Model file for the job. Use its own axes, mm. Face numbers are marked on the shaded views. A direction names the side the tool comes from. Give positions to 0.01 mm unless a question says otherwise; leave off trailing zeros. Order: outer loops, then holes, each group sorted by start corner. A loop starts at its lowest first (then second) coordinate and runs counter-clockwise, first axis right, second up. Notation, with made-up numbers: (25, 69.25) -> (68, 69.25) arc R20 ccw to (68, 92.25) -> close; hole circle Ø11 at (39.25, 86). An arc over 180 degrees is marked (long way). Answer in a Markdown table with one row per item. Add a question column.
from build123d import *

# Parameters (mm, degrees)
EXTRUDE_THIN1_DEPTH        = 12.7
FILLET1_R                  = 12.7
SKETCH2_R                  = 3.9624
CUT_EXTRUDE1_DEPTH         = 71.952548404
F_31_0_12_DIAMETER_HOLE1_D = 3.048


with BuildPart() as part:
    # Sketch1 → Extrude-Thin1 (new, symmetric)
    with BuildSketch(Plane.XY):
        with BuildLine():
            Line((-26.035, -64.77), (-26.035, -3.9624))
            ThreePointArc((-26.035, -3.9624), (-24.87443991, -1.16056009), (-22.0726, 0))
            Line((-22.0726, 0), (22.0726, 0))
            ThreePointArc((22.0726, 0), (24.87443991, -1.16056009), (26.035, -3.9624))
            Line((26.035, -3.9624), (26.035, -64.77))
            Line((26.035, -64.77), (23.876, -64.77))
            Line((23.876, -64.77), (23.876, -3.9624))
            ThreePointArc((23.876, -3.9624), (23.347796369, -2.687203631), (22.0726, -2.159))
            Line((22.0726, -2.159), (-22.0726, -2.159))
            ThreePointArc((-22.0726, -2.159), (-23.347796369, -2.687203631), (-23.876, -3.9624))
            Line((-23.876, -3.9624), (-23.876, -64.77))
            Line((-23.876, -64.77), (-26.035, -64.77))
        make_face()
    extrude(amount=EXTRUDE_THIN1_DEPTH, both=True)

    # Fillet1
    fillet1_edges = [part.edges().sort_by_distance(p)[0] for p in [
        (24.9555, -64.77, -12.7),
        (24.9555, -64.77, 12.7),
        (-24.9555, -64.77, -12.7),
        (-24.9555, -64.77, 12.7),
    ]]
    fillet(fillet1_edges, radius=FILLET1_R - 0.0001)  # a hair under: the kernel refuses the full size

    # Sketch2 → Cut-Extrude1 (cut, through all)
    with BuildSketch(Plane(origin=(0, 0, 0), x_dir=(1, 0, 0), z_dir=(0, 1, 0))):
        with Locations(Location((0, 0, 0), (0, 0, 270))):
            Circle(SKETCH2_R)
    extrude(amount=-CUT_EXTRUDE1_DEPTH, mode=Mode.SUBTRACT)

    # #31 (0.12) Diameter Hole1 (through all)
    with Locations(Plane(origin=(0, 0, 0), x_dir=(1, 0, 0), z_dir=(0, 1, 0))):
        with Locations((0, -7.112), (0, 7.112), (-7.112, 0), (7.112, 0), (18.6309, 0), (-18.6309, 0)):
            Hole(F_31_0_12_DIAMETER_HOLE1_D / 2)


solid = part.part
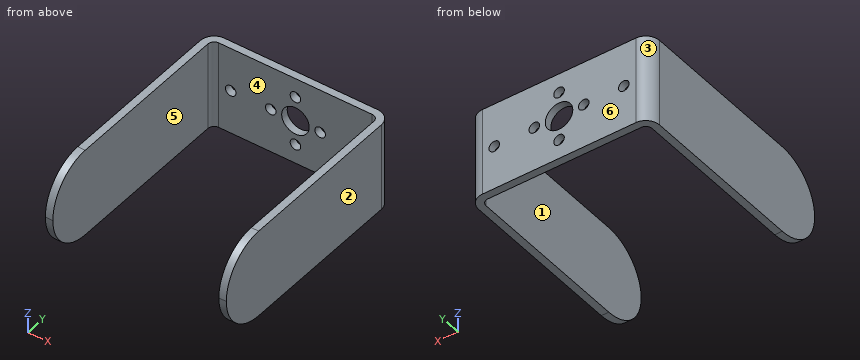
Item 1: Saw through at B-B on y = -21. List the corners of the cut face in (x, z) (3 decimals), plus the area to 3 significant figures.
Item 2: Two-plate mould, pull along X, no slides. Class the marked faces 1, 2, 3 and 4: pulls with the +X half, pulls with the -X half, needs draft (parallel to the pull), parting line crosses it, or undercut.
Item 3: Saw through at C-C on z = 10. List the corners of the cut face in (x, y) (3 decimals).
Item 4: Saw through at A-A on x = 0. List the corners of the cut face in (y, z), plus the area to 3 significant figures.
Item 5: Pin check, flat tips, straight feed: pin 1 Ø4 at (x, z) = (7.112, 0) entering from -Y; pin 2 Ø2.5 at (x, z) = (0, 7.112) entering from +Y. Stop position of each tip, or through.
Item 6: Wall check: line 1 (X direction, y = -26, z = 10.75) (3 decimals); line 2 (Y direction, x = 8.5, z = 5.5); line 3 (X direction, y = -3.5, z = 10.5). Give the ranges that are in metal, low to high.
Item 7: Which spindle directions (+Z, -Z, +X, -X, +Y, -Y) get a long thin tool onto all of the face, cutting with end or side? Do the marked faces 5 and 6. Say none if no direction does.
Evaluation:
| question | item | result |
|---|---|---|
| 1 | outline | (-26.035, -12.7) -> (-23.876, -12.7) -> (-23.876, 12.7) -> (-26.035, 12.7) -> close; (23.876, -12.7) -> (26.035, -12.7) -> (26.035, 12.7) -> (23.876, 12.7) -> close |
| 1 | area | 110 mm2 |
| 2 | face 1 | undercut |
| 2 | face 2 | pulls with the +X half |
| 2 | face 3 | pulls with the -X half |
| 2 | face 4 | undercut |
| 3 | outline | (-26.035, -59.899) -> (-23.876, -59.899) -> (-23.876, -3.962) arc R1.803 cw to (-22.073, -2.159) -> (22.073, -2.159) arc R1.803 cw to (23.876, -3.962) -> (23.876, -59.899) -> (26.035, -59.899) -> (26.035, -3.962) arc R3.962 ccw to (22.073, 0) -> (-22.073, 0) arc R3.962 ccw to (-26.035, -3.962) -> close |
| 4 | outline | (-2.16, -12.7) -> (0, -12.7) -> (0, -8.64) -> (-2.16, -8.64) -> close; (-2.16, -5.59) -> (0, -5.59) -> (0, -3.96) -> (-2.16, -3.96) -> close; (-2.16, 3.96) -> (0, 3.96) -> (0, 5.59) -> (-2.16, 5.59) -> close; (-2.16, 8.64) -> (0, 8.64) -> (0, 12.7) -> (-2.16, 12.7) -> close |
| 4 | area | 24.6 mm2 |
| 5 | pin 1 | stops at y = -2.16 |
| 5 | pin 2 | passes through |
| 6 | line 1 | x = -26.035 to -23.876, 23.876 to 26.035 |
| 6 | line 2 | y = -2.16 to 0 |
| 6 | line 3 | x = -26.01 to -23.82, 23.82 to 26.01 |
| 7 | face 5 | +Z, -Z, -Y |
| 7 | face 6 | +Z, -Z, +X, -X, +Y |
